from build123d import *

# Parameters (mm, degrees)
SKETCH1_R               = 14
BOSS_EXTRUDE1_DEPTH     = 105
SKETCH2_R               = 24
CUT_EXTRUDE1_DEPTH      = 110.567330897
SKETCH4_R               = 25
CUT_EXTRUDE2_DEPTH      = 9.4
SKETCH5_R               = 12
CUT_EXTRUDE3_DEPTH      = 123
SKETCH10_R              = 14
SKETCH8_R               = 24
SKETCH12_R              = 24
SKETCH12_R_2            = 19
BOSS_EXTRUDE2_DEPTH     = 24
SKETCH13_R              = 1.6
CUT_EXTRUDE4_DEPTH      = 8
CUT_EXTRUDE6_DEPTH      = 6
BOSS_EXTRUDE7_DEPTH     = 1
CUT_EXTRUDE7_OUTLINE_W  = 25.205591592
CUT_EXTRUDE7_OUTLINE_H  = 24
CUT_EXTRUDE7_DEPTH      = 2.781366517
SKETCH20_R              = 4
SKETCH20_R_2            = 3.5
CUT_EXTRUDE8_DEPTH      = 10
SKETCH22_R              = 1.05
BOSS_EXTRUDE8_DEPTH     = 1
CUT_EXTRUDE9_DEPTH      = 10
CUT_EXTRUDE9_DEPTH_BACK = 5
SKETCH23_R              = 2


with BuildPart() as part:
    # Sketch1 → Boss-Extrude1 (new body)
    with BuildSketch(Plane(origin=(0, 0, 0), x_dir=(1, 0, 0), z_dir=(0, 1, 0))):
        with Locations(Location((0, 0, 0), (0, 0, 270))):
            Circle(SKETCH1_R)
    extrude(amount=BOSS_EXTRUDE1_DEPTH)

    # Sketch2 → Cut-Extrude1 (cut, through all)
    with BuildSketch(Plane(origin=(0, 0, -14), x_dir=(-1, 0, 0), z_dir=(0, 0, -1))):
        with Locations((0, 105)):
            Circle(SKETCH2_R)
    extrude(amount=-CUT_EXTRUDE1_DEPTH, mode=Mode.SUBTRACT)

    # Sketch4 → Cut-Extrude2 (cut)
    with BuildSketch(Plane(origin=(0, 0, -14), x_dir=(-1, 0, 0), z_dir=(0, 0, -1))):
        with Locations((0, 105)):
            Circle(SKETCH4_R)
    extrude(amount=-CUT_EXTRUDE2_DEPTH, mode=Mode.SUBTRACT)

    # Sketch5 → Cut-Extrude3 (cut)
    with BuildSketch(Plane.XZ):
        with Locations(Location((0, 0, 0), (0, 0, 270))):
            Circle(SKETCH5_R)
    extrude(amount=-CUT_EXTRUDE3_DEPTH, mode=Mode.SUBTRACT)

    # Sketch10 → Loft6 section 0
    with BuildSketch(Plane(origin=(0, 0, 0), x_dir=(-1, 0, 0), z_dir=(0, -1, 0))):
        Circle(SKETCH10_R)
    # Sketch8 → Loft6 section 1
    with BuildSketch(Plane(origin=(0, -5, 0), x_dir=(-1, 0, 0), z_dir=(0, -1, 0))):
        Circle(SKETCH8_R)
    loft()

    # Cut-Loft1: read off the stored shape, not the designer's step
    # Cut-Loft1: loft between two sections, ruled curve by curve
    cut_loft1_from = [
        Edge.make_bspline([(-6.918556866, 0, -9.804772863), (12.69098886, 0, -23.641886595), (26.528102592, 0, -4.032340869), (6.918556866, 0, 9.804772863), (-12.69098886, 0, 23.641886595), (-26.528102592, 0, 4.032340869), (-6.918556866, 0, -9.804772863)], [0, 0, 0, 0, 0.5, 0.5, 0.5, 1, 1, 1, 1], 3, [1, 0.333333333, 0.333333333, 1, 0.333333333, 0.333333333, 1]),
    ]
    cut_loft1_to = [
        Edge.make_bspline([(3.659825819, -5, -21.693447743), (47.046721305, -5, -14.373796105), (39.727069667, -5, 29.013099381), (-3.659825819, -5, 21.693447743), (-47.046721305, -5, 14.373796105), (-39.727069667, -5, -29.013099381), (3.659825819, -5, -21.693447743)], [0, 0, 0, 0, 0.5, 0.5, 0.5, 1, 1, 1, 1], 3, [1, 0.333333333, 0.333333333, 1, 0.333333333, 0.333333333, 1]),
    ]
    cut_loft1 = Solid(Shell([*[Face.make_surface_from_curves(cut_loft1_from[k], cut_loft1_to[k]) for k in range(1)], Face(Wire(cut_loft1_from)), Face(Wire(cut_loft1_to))]))
    add(cut_loft1, mode=Mode.SUBTRACT)

    # Sketch12 → Boss-Extrude2 (add)
    with BuildSketch(Plane.XZ.offset(5)):
        Circle(SKETCH12_R)
        Circle(SKETCH12_R_2, mode=Mode.SUBTRACT)
    extrude(amount=BOSS_EXTRUDE2_DEPTH)

    # Sketch13 → Cut-Extrude4 (cut)
    with BuildSketch(Plane.XZ.offset(29)):
        with Locations(Location((-15.202795796, 15.202795796, 0), (0, 0, 270))):
            Circle(SKETCH13_R)
        with Locations(Location((15.202795796, 15.202795796, 0), (0, 0, 270))):
            Circle(SKETCH13_R)
        with Locations(Location((15.202795796, -15.202795796, 0), (0, 0, 270))):
            Circle(SKETCH13_R)
        with Locations(Location((-15.202795796, -15.202795796, 0), (0, 0, 270))):
            Circle(SKETCH13_R)
    extrude(amount=-CUT_EXTRUDE4_DEPTH, mode=Mode.SUBTRACT)

    # Sketch15 → Cut-Extrude6 (cut)
    with BuildSketch(Plane.XY.offset(24)):
        Polygon((-24, -5), (-24, -29), (24, -29), (24, -5), (14, 0), (-14, 0), align=None)
    extrude(amount=-CUT_EXTRUDE6_DEPTH, mode=Mode.SUBTRACT)

    # Sketch17 → Boss-Extrude7 (add)
    with BuildSketch(Plane.XY.offset(18)):
        with BuildLine():
            Line((15.874507866, -29), (15.874507866, -5))
            add(Edge.make_bspline(
                [(-15.874507866, -5), (-14.594943965, -4.576824016), (-12.019648156, -3.781972699), (-9.397994136, -3.134788187), (-7.407221822, -2.727541998), (-6.739521939, -2.6048822), (-5.394539357, -2.390087157), (-4.71546375, -2.297841059), (-2.684830415, -2.075564646), (-1.33504572, -1.999607533), (1.356128498, -2.000395553), (2.697521645, -2.07707476), (5.372653744, -2.369657545), (6.706415867, -2.585139688), (8.702458542, -2.992042885), (9.36832807, -3.141896909), (10.69006115, -3.463557333), (11.346413002, -3.635391758), (13.304203001, -4.178353981), (14.594485661, -4.576672447), (15.874507866, -5)],
                knots=[0, 0, 0, 0, 0.125, 0.25, 0.25, 0.3125, 0.3125, 0.375, 0.375, 0.5, 0.5, 0.625, 0.625, 0.75, 0.75, 0.8125, 0.8125, 0.875, 0.875, 1, 1, 1, 1], degree=3))
            Line((-15.874507866, -5), (-15.874507866, -29))
            Line((-15.874507866, -29), (15.874507866, -29))
        make_face()
    extrude(amount=-BOSS_EXTRUDE7_DEPTH)

    # Cut-Extrude7: read off the stored shape, not the designer's step
    # Cut-Extrude7 outline → Cut-Extrude7 (cut)
    with BuildSketch(Plane(origin=(0, 0, 17), x_dir=(-1, 0, 0), z_dir=(0, 0, -1))):
        with Locations((0, -17)):
            Rectangle(CUT_EXTRUDE7_OUTLINE_W, CUT_EXTRUDE7_OUTLINE_H)
    extrude(amount=CUT_EXTRUDE7_DEPTH, mode=Mode.SUBTRACT)

    # Sketch20 → Cut-Extrude8 (cut)
    with BuildSketch(Plane.XY.offset(18)):
        with Locations((6.602795796, -10)):
            Circle(SKETCH20_R)
        with Locations((-6.602795796, -10)):
            Circle(SKETCH20_R_2)
    extrude(amount=-CUT_EXTRUDE8_DEPTH, mode=Mode.SUBTRACT)

    # Sketch23 → Cut-Extrude9 (cut, two sides: drawn at the far end of the back side and taken through both)
    with BuildSketch(Plane.XY.offset(-12).offset(-CUT_EXTRUDE9_DEPTH_BACK)):
        with Locations(Location((0, 4, 0), (0, 0, 90))):
            Circle(SKETCH23_R)
    extrude(amount=CUT_EXTRUDE9_DEPTH + CUT_EXTRUDE9_DEPTH_BACK, mode=Mode.SUBTRACT)


with BuildPart() as body_2:
    # Sketch22 → Boss-Extrude8 (new body)
    with BuildSketch(Plane.XZ.offset(29)):
        with BuildLine():
            Line((-15.874507866, 18), (15.874507866, 18))
            ThreePointArc((15.874507866, 18), (0, -24), (-15.874507866, 18))
        make_face()
        with Locations(Location((-15.202795796, 15.202795796, 0), (0, 0, 270))):
            Circle(SKETCH22_R, mode=Mode.SUBTRACT)
        with Locations(Location((15.202795796, 15.202795796, 0), (0, 0, 270))):
            Circle(SKETCH22_R, mode=Mode.SUBTRACT)
        with Locations(Location((15.202795796, -15.202795796, 0), (0, 0, 270))):
            Circle(SKETCH22_R, mode=Mode.SUBTRACT)
        with Locations(Location((-15.202795796, -15.202795796, 0), (0, 0, 270))):
            Circle(SKETCH22_R, mode=Mode.SUBTRACT)
    extrude(amount=BOSS_EXTRUDE8_DEPTH)


solid = part.part
Verification items for the finished model (mm, model axes). A direction names the side the tool comes from. Coordinates: 2 decimals unless noted, no trailing zeros. Write each loop counter-clockwise with the first axis right and the second up, starting at its lowest first coordinate (ties: lowest second). Pieces come first, ordered by that corner, then holes. Notation, with made-up numbers: M 23,68 L 46,68 A27 ccw 46,84 Z; hole C 3,-25.5 d7. An arc over 180 degrees is marked long. One line per question, with ' | ' between items.
1) Release check for a two-part mould opening along Z. For faces 5 (the face through (-12.603, -17, 16)), 6 (the face through (8.45, -13.55, 17.51)), 7 (the face through (-5.362, 42.155, 12.932)) record: +Z half, -Z half, draft (parallel to the pull), parting line (faces both ways), or undercut.
Solutions:
face 5: undercut | face 6: draft | face 7: parting line
2) Sectioned sample at C-C on y = 4. Record the cut outline in (x, z), then the cut area to 3 significant figures.
Solutions:
outline: M -2,-13.86 L -2,-11.83 A12 cw long 2,-11.83 L 2,-13.86 A14 ccw long Z | area: 155 mm^2
3) Sectioned sample at B-B on y = 16. Record the cut outline in (x, z).
Solutions:
outline: C 0,0 d28; hole C 0,0 d24
4) Depth check by flat-ended pin: pin 1 Ø0.8 at (y, z) = (-12.5, 16) entering from -X; pin 2 Ø3 at (x, z) = (-15.2, -15.2) entering from -Y; pin 3 Ø1.1 at (x, y) = (12, 84.5) entering from -Z; pin 4 Ø10 at (x, z) = (16.5, 4.5) entering from -Y. Enter the tip coordinate at first touch or a pass-through.
Solutions:
pin 1: x = -18.24 | pin 2: y = -21 | pin 3: z = -4.6 | pin 4: y = -29
5) Access from +Z, -Z, +X, -X, +Y, -Y to the whole of each face (thin tool, end or side, straight path). Record for faces 1 (the face through (1.097, 80.024, -12.108)), 2 (the face through (5, -5, -19)), 3 (the face through (12.603, -17, 16)), 4 (the face through (-1.352, 2.526, -12.931)).
Solutions:
face 1: -Z, +Y | face 2: none | face 3: -Y | face 4: -Z
6) Sectioned sample at A-A on y = -10. Record the cut outline in (x, z), then the cut area to 3 significant figures.
Solutions:
outline: M -15.87,18 A24 ccw long 15.87,18 L 10.6,18 L 10.6,17 L 12.6,17 L 12.6,14.22 A19 cw long -12.6,14.22 L -12.6,17 L -10.1,17 L -10.1,18 Z; M -3.1,17 L 2.6,17 L 2.6,18 L -3.1,18 Z | area: 542 mm^2
7) Material ranges on L1, parallel to Z at x = 0, y = 21; L2, parallel to X at y = 64, z = -8; L3, parallel to Z at x = 9, y = 74, recorded low to high.
Solutions:
L1: -14 to -12, 12 to 14 | L2: -11.49 to -8.94, 8.94 to 11.49 | L3: -10.72 to -7.94, 7.94 to 10.72
